```python
from build123d import *

# Parameters (mm, degrees)
F0_R     = 57.15
F1_DEPTH = 12.7
F2_R     = 82.073796
F2_R_2   = 48.26
F3_DEPTH = 1.5875
F4_SIZE  = 4.7625


with BuildPart() as f1:
    # F0 (on Top) → F1 (new body)
    with BuildSketch(Plane.XY):
        Circle(F0_R)
    extrude(amount=F1_DEPTH)

    # F2 (on face) → F3 (cut)
    with BuildSketch(Plane.XY.offset(12.7)):
        Circle(F2_R)
        Circle(F2_R_2, mode=Mode.SUBTRACT)
    extrude(amount=-F3_DEPTH, mode=Mode.SUBTRACT)

    # F4
    f4_edges = [f1.edges().sort_by_distance(p)[0] for p in [
        (-57.15, 0, 11.1125),
    ]]
    chamfer(f4_edges, length=F4_SIZE)


solid = f1.part
```
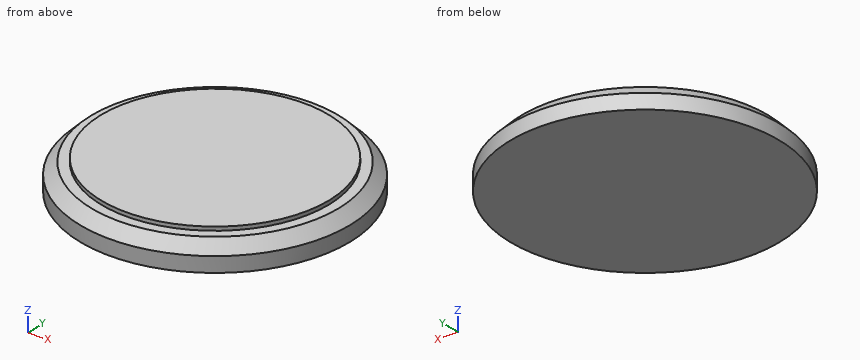
Source: CAD feature listing. Evaluate the final solid. Frame: model axes, mm. Coordinates: 2 decimals unless noted, no trailing zeros. Order: outer loops, then holes, each group sorted by start corner. A loop starts at its lowest first (then second) coordinate and runs counter-clockwise, first axis right, second up. Notation, with made-up numbers: M 40.5,-16.5 L 86.5,-16.5 A14 cw 86.5,-12.5 Z; hole C 77.5,42 d6. An arc over 180 degrees is marked long. Write each question's results on one line, items separated by ' | '. Start each with the question number.
1) Line query: line 1 (Z direction, x = 10, y = -47.5); line 2 (Y direction, x = -3, z = 7.5); line 3 (X direction, y = 28.5, z = 1.25). Output: solid intervals per line, ascending. Write a range as from..to.
2) Section query C-C (z = 5). Return the cut outline in (x, y).
3) Contact query for flat-ended pins moving along their axis: pin 1 Ø1.5 at (x, z) = (22, 11) entering from +Y; pin 2 Ø4 at (y, z) = (-14.5, 8.5) entering from -X; pin 3 Ø1 at (x, z) = (-34.5, 11) entering from -Y. Output: stop coordinate, or through.
4) Section query A-A (y = 0). Return the cut outline in (x, z).
Answers:
1) line 1: z = 0..11.11 | line 2: y = -55.92..55.92 | line 3: x = -49.54..49.54
2) outline: C 0,0 d114.3
3) pin 1: stops at y = 48.56 | pin 2: stops at x = -55.19 | pin 3: stops at y = -40.36
4) outline: M -57.15,0 L 57.15,0 L 57.15,6.35 L 52.39,11.11 L 48.26,11.11 L 48.26,12.7 L -48.26,12.7 L -48.26,11.11 L -52.39,11.11 L -57.15,6.35 Z
